Input: dimensioned drawing with shaded views. Units: mm. Origin: part minimum x, y, z. Round coordinates to 2 decimals unless told otherwise and drop trailing zeros. Loops run counter-clockwise (first coordinate to the right, second up) from the corner with the lowest first, then second, coordinate; pieces in that order, holes last. Notation, with made-up numbers: (53.5, 18) - (77.5, 18) arc R11 cw to (77.5, 25) - close; hole circle Ø8 at (13, -27). An arc over 180 degrees is marked (long way). One line per question, with ' | ' between items. Start each with the question number.
1. Cut plane D-D (z = 22.5). Return loops of the section in (x, y), then the cut area to 3 significant figures.
2. Ray query, line 1 (X direction, y = 4.25, z = 59.5); line 2 (Y direction, x = 4.5, z = 53.5); line 3 (Z direction, x = 8, y = 3). Return the intervals inside material, ascending.
3. Cut plane C-C (z = 57.5). Return loops of the section in (x, y).
4. Mould query, pull axis Y, two halves, no side actions, for the marked faces 1 and 2. Classes: pulls with the +Y half, pulls with the -Y half, needs draft (parallel to the pull), parting line crosses it, or undercut.
5. Cut plane A-A (x = 4.25). Return loops of the section in (y, z), then the cut area to 4 significant figures.
6. Pin query (flat end, axial travel): pin 1 (3 mm diameter, centred on y = 3, z = 55, fed in from -X); pin 2 (1 mm diameter, centred on x = 6.5, z = 17.5, fed in from -Y); pin 3 (2 mm diameter, centred on x = 4.5, y = 4, fed in from +Z); pin 4 (2 mm diameter, centred on x = 2, z = 21.5, fed in from +Y). Return the tip coordinate at first contact, or that it passes through.
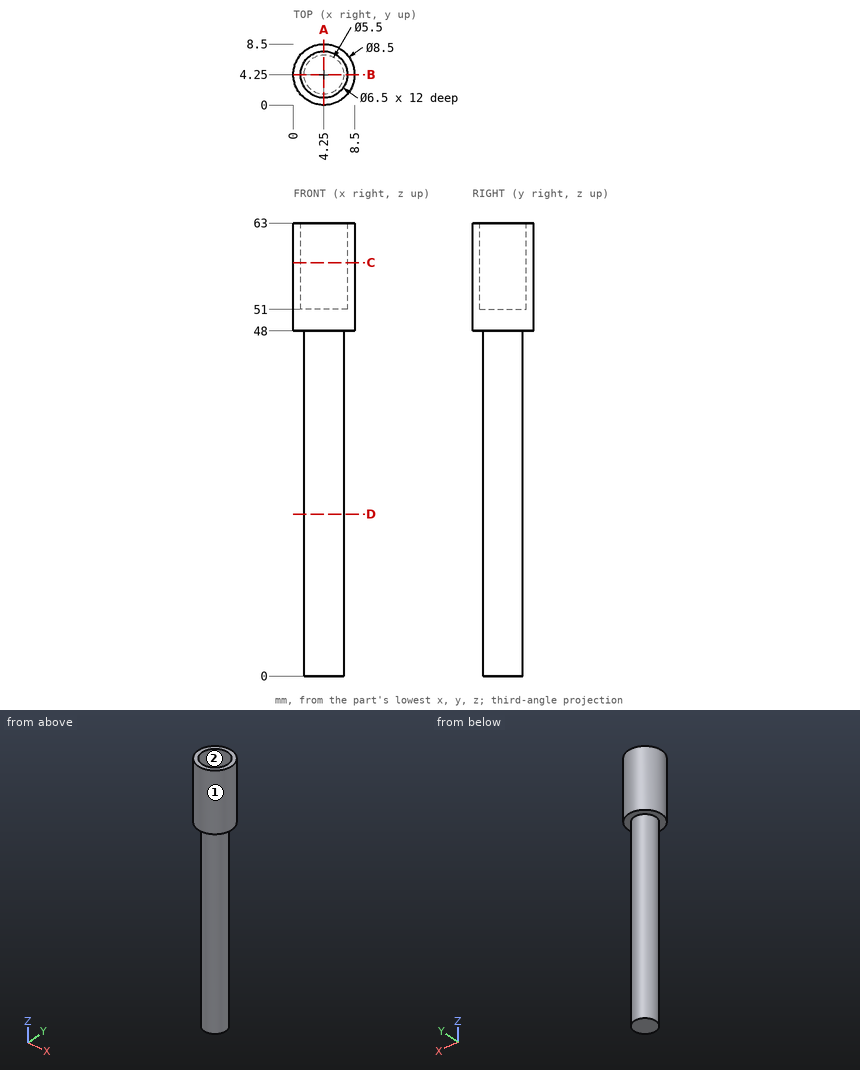
Answers follow:
1) outline: circle Ø5.5 at (4.25, 4.25) | area: 23.8 mm2
2) line 1: x = 0 to 1, 7.5 to 8.5 | line 2: y = 0.01 to 1.01, 7.49 to 8.49 | line 3: z = 48 to 63
3) outline: circle Ø8.5 at (4.25, 4.25); hole circle Ø6.5 at (4.25, 4.25)
4) face 1: parting line crosses it | face 2: undercut
5) outline: (0, 48) - (1.5, 48) - (1.5, 0) - (7, 0) - (7, 48) - (8.5, 48) - (8.5, 63) - (7.5, 63) - (7.5, 51) - (1, 51) - (1, 63) - (0, 63) - close | area: 313.5 mm2
6) pin 1: stops at x = 0 | pin 2: stops at y = 2.13 | pin 3: stops at z = 51 | pin 4: stops at y = 6.7
